Verification items for the finished model (mm, model axes). Give positions to 0.01 mm unless a question says otherwise; leave off trailing zeros. Write each loop counter-clockwise with the first axis right and the second up, starting at its lowest first coordinate (ties: lowest second). Pieces come first, ordered by that corner, then holes. Notation, with made-up numbers: M -34.5,77 L -20.5,77 A32 ccw -20.5,104 Z; hole C 6.25,50 d10. An arc over 180 degrees is marked long. Write item = value, one per line.
from build123d import *

# Parameters (mm, degrees)
F0_R     = 522.5
F1_DEPTH = 3.18


with BuildPart() as f1:
    # F0 (on Top) → F1 (new body)
    with BuildSketch(Plane.XY):
        Circle(F0_R)
        with BuildLine():
            ThreePointArc((456.846254, 78.55), (461.871023, 39.417771), (463.55, 0))
            ThreePointArc((463.55, 0), (461.831965, -39.872779), (456.690595, -79.45))
            ThreePointArc((456.690595, -79.45), (456.158203, -82.451783), (455.60608, -85.45))
            ThreePointArc((455.60608, -85.45), (426.442242, -181.729515), (377.193982, -269.45))
            ThreePointArc((377.193982, -269.45), (375.026465, -272.458718), (372.83495, -275.45))
            ThreePointArc((372.83495, -275.45), (0, -463.55), (-372.83495, -275.45))
            ThreePointArc((-372.83495, -275.45), (-375.026465, -272.458718), (-377.193982, -269.45))
            ThreePointArc((-377.193982, -269.45), (-426.442242, -181.729515), (-455.60608, -85.45))
            ThreePointArc((-455.60608, -85.45), (-456.158203, -82.451783), (-456.690595, -79.45))
            ThreePointArc((-456.690595, -79.45), (-463.549775, -0.456681), (-456.846254, 78.55))
            ThreePointArc((-456.846254, 78.55), (-456.319967, 81.551762), (-455.773957, 84.55))
            ThreePointArc((-455.773957, 84.55), (-426.837312, 180.799645), (-377.835282, 268.55))
            ThreePointArc((-377.835282, 268.55), (-375.678716, 271.558659), (-373.498193, 274.55))
            ThreePointArc((-373.498193, 274.55), (0, 463.55), (373.498193, 274.55))
            ThreePointArc((373.498193, 274.55), (375.678716, 271.558659), (377.835282, 268.55))
            ThreePointArc((377.835282, 268.55), (426.837312, 180.799645), (455.773957, 84.55))
            ThreePointArc((455.773957, 84.55), (456.319967, 81.551762), (456.846254, 78.55))
        make_face(mode=Mode.SUBTRACT)
        with BuildLine():
            Line((-377.835282, 268.55), (377.835282, 268.55))
            ThreePointArc((377.835282, 268.55), (375.678716, 271.558659), (373.498193, 274.55))
            Line((373.498193, 274.55), (-373.498193, 274.55))
            ThreePointArc((-373.498193, 274.55), (-375.678716, 271.558659), (-377.835282, 268.55))
        make_face()
        with BuildLine():
            Line((-456.846254, 78.55), (456.846254, 78.55))
            ThreePointArc((456.846254, 78.55), (456.319967, 81.551762), (455.773957, 84.55))
            Line((455.773957, 84.55), (-455.773957, 84.55))
            ThreePointArc((-455.773957, 84.55), (-456.319967, 81.551762), (-456.846254, 78.55))
        make_face()
        with BuildLine():
            ThreePointArc((455.60608, -85.45), (456.158203, -82.451783), (456.690595, -79.45))
            Line((456.690595, -79.45), (-456.690595, -79.45))
            ThreePointArc((-456.690595, -79.45), (-456.158203, -82.451783), (-455.60608, -85.45))
            Line((-455.60608, -85.45), (455.60608, -85.45))
        make_face()
        with BuildLine():
            ThreePointArc((372.83495, -275.45), (375.026465, -272.458718), (377.193982, -269.45))
            Line((377.193982, -269.45), (-377.193982, -269.45))
            ThreePointArc((-377.193982, -269.45), (-375.026465, -272.458718), (-372.83495, -275.45))
            Line((-372.83495, -275.45), (372.83495, -275.45))
        make_face()
    extrude(amount=F1_DEPTH)


solid = f1.part
1) Depth check by flat-ended pin: P1, Ø1, axis at x = -102, z = 2, coming from the +Y side; P2, Ø1.6, axis at x = 42.5, z = 2, coming from the -Y side; P3, Ø1, axis at y = 354.5, z = 1.5, coming from the +X side. Enter the tip coordinate at first touch or a pass-through.
From the geometry:
P1 = 512.55
P2 = -520.83
P3 = 384.3
2) Cross-section at D-D on x = -403. Record the boundary of the cut face in (y, z), plus the area to 3 significant figures.
From the geometry:
outline = M -332.56,0 L -229.06,0 L -229.06,3.18 L -332.56,3.18 Z; M -85.45,0 L -79.45,0 L -79.45,3.18 L -85.45,3.18 Z; M 78.55,0 L 84.55,0 L 84.55,3.18 L 78.55,3.18 Z; M 229.06,0 L 332.56,0 L 332.56,3.18 L 229.06,3.18 Z
area = 696 mm^2
3) Cross-section at C-C on y = -393. Record the boundary of the cut face in (x, z).
From the geometry:
outline = M -344.32,0 L -245.82,0 L -245.82,3.18 L -344.32,3.18 Z; M 245.82,0 L 344.32,0 L 344.32,3.18 L 245.82,3.18 Z
4) Draft check along X on faces 1 (the cylindrical face through (498.372, 156.945, 1.568)), 2 (the flat face through (-41, 80, 3.18)), 3 (the cylindrical face through (426.993, -180.43, 1.568)). Enter one of: +X half, -X half, draft (parallel to the pull), parting line (faces both ways), or undercut.
From the geometry:
face_1 = parting line
face_2 = draft
face_3 = undercut
5) Material ranges on probe 1 along Y at (x, z) = (393.5, 0.7); probe 2 along Y at (x, z) = (-225, 1.05); probe 3 along Y at (x, z) = (255, 2.8), recorded low to high. Write a range as from..to.
From the geometry:
probe_1 = -343.75..-245.02, -85.45..-79.45, 78.55..84.55, 245.02..343.75
probe_2 = -471.57..-405.28, -275.45..-269.45, -85.45..-79.45, 78.55..84.55, 268.55..274.55, 405.28..471.57
probe_3 = -456.05..-387.11, -275.45..-269.45, -85.45..-79.45, 78.55..84.55, 268.55..274.55, 387.11..456.05
6) Cross-section at A-A on z = 2.3. Record the boundary of the cut face in (x, y).
From the geometry:
outline = C 0,0 d1045; hole M -456.85,78.55 A463.55 ccw -456.69,-79.45 L 456.69,-79.45 A463.55 ccw 463.55,0 A463.55 ccw 456.85,78.55 Z; hole M -455.77,84.55 L 455.77,84.55 A463.55 ccw 377.84,268.55 L -377.84,268.55 A463.55 ccw Z; hole M -455.61,-85.45 A463.55 ccw -377.19,-269.45 L 377.19,-269.45 A463.55 ccw 455.61,-85.45 Z; hole M -373.5,274.55 L 373.5,274.55 A463.55 ccw Z; hole M -372.83,-275.45 A463.55 ccw 372.83,-275.45 Z
7) Cross-section at B-B on x = 0. Record the boundary of the cut face in (y, z), plus the area to 3 significant figures.
From the geometry:
outline = M -522.5,0 L -463.55,0 L -463.55,3.18 L -522.5,3.18 Z; M -275.45,0 L -269.45,0 L -269.45,3.18 L -275.45,3.18 Z; M -85.45,0 L -79.45,0 L -79.45,3.18 L -85.45,3.18 Z; M 78.55,0 L 84.55,0 L 84.55,3.18 L 78.55,3.18 Z; M 268.55,0 L 274.55,0 L 274.55,3.18 L 268.55,3.18 Z; M 463.55,0 L 522.5,0 L 522.5,3.18 L 463.55,3.18 Z
area = 451 mm^2
